Design review of the part built by this model. Coordinates are the model's own, in mm. A direction names the side the tool comes from. Coordinates: 2 decimals unless noted, no trailing zeros. Write each loop counter-clockwise with the first axis right and the second up, starting at its lowest first coordinate (ties: lowest second). Pieces come first, ordered by that corner, then holes. Notation, with made-up numbers: M 52,30 L 81,30 A16 cw 81,46 Z; hole C -39,82.5 d9. An arc over 180 degrees is marked long. Write item = value, one per line.
```python
from build123d import *

# Parameters (mm, degrees)
SKETCH1_R                       = 5
BOSS_EXTRUDE1_DEPTH             = 20
SKETCH2_R                       = 10.033
BOSS_EXTRUDE2_DEPTH             = 38.1
F_5_0MM_DOWEL_HOLE1_D           = 5
F_5_0MM_DOWEL_HOLE1_CSINK_D     = 5.05
F_5_0MM_DOWEL_HOLE1_CSINK_ANGLE = 90


with BuildPart() as part:
    # Sketch1 → Boss-Extrude1 (new body)
    with BuildSketch(Plane.XY):
        Circle(SKETCH1_R)
    extrude(amount=BOSS_EXTRUDE1_DEPTH)

    # Sketch2 → Boss-Extrude2 (add)
    with BuildSketch(Plane.XY.offset(20)):
        with Locations(Location((0, 0, 0), (0, 0, 180))):
            Circle(SKETCH2_R)
    extrude(amount=BOSS_EXTRUDE2_DEPTH)

    # Ø5.0mm Dowel Hole1 (through all)
    with Locations(Plane(origin=(0, 10.033, 0), x_dir=(1, 0, 0), z_dir=(0, 1, 0))):
        with Locations((0, -6), (0, -39.05)):
            CounterSinkHole(F_5_0MM_DOWEL_HOLE1_D / 2, F_5_0MM_DOWEL_HOLE1_CSINK_D / 2, counter_sink_angle=F_5_0MM_DOWEL_HOLE1_CSINK_ANGLE)


solid = part.part
```
Q1. Consider section B-B, the plane y = 0. State the section outline as (x, z) points, and give its area (3 significant figures).
Check result:
outline = M -10.03,20 L -5,20 L -5,0 L 5,0 L 5,20 L 10.03,20 L 10.03,58.1 L -10.03,58.1 Z; hole C 0,6 d5; hole C 0,39.05 d5
area = 925 mm²
Q2. The part is to be moulded in two halves that separate along X. For faces 3 (the cylindrical face through (-9.57, -3.01, 38.78)), 4 (the cylindrical face through (-2.385, -0.07, 5.249)), 5 (the flat face through (5, 2, 20)), say which applies: +X half, -X half, draft (parallel to the pull), parting line (faces both ways), or undercut.
Check result:
face_3 = parting line
face_4 = undercut
face_5 = draft
Q3. Consider section C-C, the plane z = 19. State the section outline as (x, y) points.
Check result:
outline = C 0,0 d10
Q4. Consider section D-D, the plane x = 3.75. State the section outline as (y, z) points.
Check result:
outline = M -9.31,20 L -3.31,20 L -3.31,0 L 3.31,0 L 3.31,20 L 9.31,20 L 9.31,58.1 L -9.31,58.1 Z
Q5. Wall thickness on line 1 (Z direction, x = 0.25, y = -0.75); line 2 (Z direction, x = 0.75, y = -5.5); line 3 (Z direction, x = -2, y = 2.25): over which ranges is each line inside the solid? List them lowest first.
Check result:
line_1 = 0 to 3.51, 8.49 to 36.56, 41.54 to 58.1
line_2 = 20 to 36.67, 41.43 to 58.1
line_3 = 0 to 4.5, 7.5 to 37.55, 40.55 to 58.1
Q6. Consider section A-A, the plane x = 0. State the section outline as (y, z) points (3 decimals), and give its area (3 significant figures).
Check result:
outline = M -10.033,20 L -5,20 L -5,8.5 L 5,8.5 L 5,20 L 10.033,20 L 10.033,36.525 L 10.008,36.55 L -10.033,36.55 Z; M -10.033,41.55 L 10.008,41.55 L 10.033,41.575 L 10.033,58.1 L -10.033,58.1 Z; M -5,0 L 5,0 L 5,3.5 L -5,3.5 Z
area = 814 mm²
Q7. Machinability: for faces 1 (the flat face through (0, 0, 58.1)), 2 (the cylindrical face through (3, 4, 10)), which of the approach directions +Z, -Z, +X, -X, +Y, -Y give a long, thin tool a straight path to every point of the face, cutting with its end or side? Answer none if there is none.
Check result:
face_1 = +Z, +X, -X, +Y, -Y
face_2 = -Z
Q8. For P1, Ø1, axis at y = 1, z = 22.5, coming from the -X side; P2, Ø4, axis at x = 4.5, z = 22, coming from the +Y side; P3, Ø3, axis at x = 0, z = 6, coming from the -Y side; P4, Ø1.5, axis at x = 7, z = 31.5, coming from the -Y side, all flat-tipped, find the tip position at first contact; note any pin that passes through.
Check result:
P1 = -10.02
P2 = 9.72
P3 = through
P4 = -7.85
